Source: CAD feature listing. Evaluate the final solid. Frame: model axes, mm. A direction names the side the tool comes from. Coordinates: 2 decimals unless noted, no trailing zeros. Order: outer loops, then holes, each group sorted by start corner. A loop starts at its lowest first (then second) coordinate and runs counter-clockwise, first axis right, second up.
```python
from build123d import *

# Parameters (mm, degrees)
BOSS_EXTRUDE1_DEPTH = 20
SKETCH2_R           = 7
SKETCH2_R_2         = 3
BOSS_EXTRUDE2_DEPTH = 5
SKETCH3_W           = 30
SKETCH3_H           = 14
SKETCH3_R           = 7
SKETCH3_R_2         = 3.5
BOSS_EXTRUDE3_DEPTH = 5


with BuildPart() as part:
    # Sketch1 → Boss-Extrude1 (new body)
    with BuildSketch(Plane.XY):
        Polygon((0, 0), (40, 0), (40, 65), (27.320508076, 65), (10, 35), (10, 14), (0, 14), align=None)
    extrude(amount=BOSS_EXTRUDE1_DEPTH)

    # Sketch2 → Boss-Extrude2 (add)
    # profile 1 of 3: a face of its own
    with BuildSketch(Plane.XY.offset(20)):
        Polygon((40, 65), (27.320508076, 65), (27.320508076, 29.29250995), (40, 35.205054136), align=None)
    # profile 2 of 3: a face of its own
    with BuildSketch(Plane.XY.offset(20)):
        with BuildLine():
            Line((72.320508076, 65), (40, 65))
            Line((40, 65), (40, 35.205054136))
            Line((40, 35.205054136), (75.278835908, 51.655845491))
            ThreePointArc((75.278835908, 51.655845491), (65.486436026, 56.484922702), (72.320508076, 65))
        make_face()
    # profile 3 of 3: a face of its own
    with BuildSketch(Plane.XY.offset(20)):
        with Locations((72.320508076, 58)):
            Circle(SKETCH2_R)
        with Locations((72.320508076, 58)):
            Circle(SKETCH2_R_2, mode=Mode.SUBTRACT)
    extrude(amount=BOSS_EXTRUDE2_DEPTH)

    # Sketch3 → Boss-Extrude3 (add)
    # profile 1 of 3: a face of its own
    with BuildSketch(Plane(origin=(0, 0, 0), x_dir=(-1, 0, 0), z_dir=(0, 0, -1))):
        with BuildLine():
            Line((-40, 0), (-40, 14))
            Line((-40, 14), (-65, 14))
            ThreePointArc((-65, 14), (-60.050252532, 11.949747468), (-58, 7))
            ThreePointArc((-58, 7), (-60.050252532, 2.050252532), (-65, 0))
            Line((-65, 0), (-40, 0))
        make_face()
    # profile 2 of 3: a face of its own
    with BuildSketch(Plane(origin=(0, 0, 0), x_dir=(-1, 0, 0), z_dir=(0, 0, -1))):
        with Locations((-25, 7)):
            Rectangle(SKETCH3_W, SKETCH3_H)
    # profile 3 of 3: a face of its own
    with BuildSketch(Plane(origin=(0, 0, 0), x_dir=(-1, 0, 0), z_dir=(0, 0, -1))):
        with Locations((-65, 7)):
            Circle(SKETCH3_R)
        with Locations((-65, 7)):
            Circle(SKETCH3_R_2, mode=Mode.SUBTRACT)
    extrude(amount=BOSS_EXTRUDE3_DEPTH)


solid = part.part
```
1. Draft query along X for faces 6 (the face through (79.18, 59.39, 22.46)), 7 (the face through (5, 14, 10)), 8 (the face through (68.497, 7.154, -2.465)). Return one class per face: released by +X, released by -X, zero draft, split by the parting line, or undercut.
Findings:
face 6: released by +X
face 7: zero draft
face 8: undercut
2. Pin query (flat end, axial travel): P1, Ø12, axis at x = 12.5, y = 21, coming from the +Z side; P2, Ø1.5, axis at y = 43.5, z = 23, coming from the -X side; P3, Ø12, axis at y = 53, z = 10.5, coming from the -X side. Return the tip coordinate at first contact, or that it passes through.
Findings:
P1: stops at z = 20
P2: stops at x = 27.32
P3: stops at x = 16.93
3. Access query for faces 1 (the face through (10, 7, -2)), 2 (the face through (37, 14, -2)), 3 (the face through (56, 7, 0)), 4 (the face through (40, 32, 10)), 5 (the face through (27.321, 47, 22)). Directions: +Z, -Z, +X, -X, +Y, -Y. A direction counts if a zero-diameter tool reaches every point of the face in a straight line with its end or side. Return the directions, or none.
Findings:
face 1: -Z, -X, +Y, -Y
face 2: -Z, +X, -X, +Y
face 3: +Z, +X, +Y, -Y
face 4: +X, +Y, -Y
face 5: +Z, -X, +Y, -Y
4. Section query D-D on y = 45.5. Return loops of the section in (x, z).
Findings:
outline: (16.06, 0) - (40, 0) - (40, 20) - (62.08, 20) - (62.08, 25) - (27.32, 25) - (27.32, 20) - (16.06, 20) - close
5. Section query A-A on y = 7. Return loops of the section in (x, z), plus the area to 4 significant figures.
Findings:
outline: (0, 0) - (10, 0) - (10, -5) - (61.5, -5) - (61.5, 0) - (40, 0) - (40, 20) - (0, 20) - close; (68.5, -5) - (72, -5) - (72, 0) - (68.5, 0) - close
area: 1,075 mm2
6. Section query C-C on z = 18.75. Return loops of the section in (x, y), plus the area to 3 significant figures.
Findings:
outline: (0, 0) - (40, 0) - (40, 65) - (27.32, 65) - (10, 35) - (10, 14) - (0, 14) - close
area: 1,830 mm2
7. Section query B-B on x = 49. Return loops of the section in (y, z).
Findings:
outline: (0, -5) - (14, -5) - (14, 0) - (0, 0) - close; (39.4, 20) - (65, 20) - (65, 25) - (39.4, 25) - close
8. Ray query, line 1 (Y direction, x = 65, z = -2.4); line 2 (X direction, y = 5, z = 4); line 3 (Z direction, x = 34.5, y = 3). Return the intervals inside material, ascending.
Findings:
line 1: y = 0 to 3.5, 10.5 to 14
line 2: x = 0 to 40
line 3: z = -5 to 20
